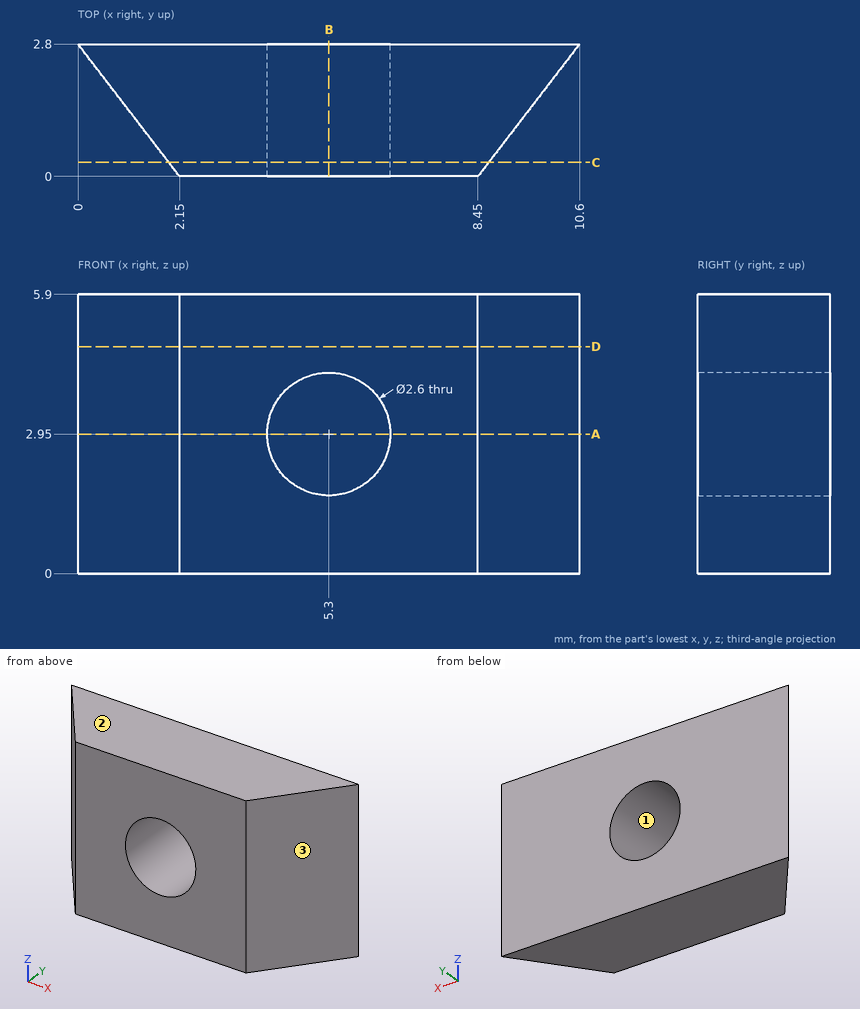
Geometry check sheet. Reference: drawing and pictorial views, mm from the part's lowest x, y, z. Coordinates: 2 decimals unless noted, no trailing zeros. Order: outer loops, then holes, each group sorted by start corner. A loop starts at its lowest first (then second) coordinate and runs counter-clockwise, first axis right, second up. Notation, with made-up numbers: (-10.5, -14.75) - (9.5, -14.75) arc R20 cw to (9.5, -6.75) - close; hole circle Ø2 at (40.25, 47). An arc over 180 degrees is marked (long way). Answer in a Markdown table with one row per item. Add a question column.
1) Cross-section at D-D, the plane z = 4.8. Record the cut outline in (x, y), then the cut area to 3 significant figures.
2) Cross-section at B-B, the plane x = 5.3. Record the cut outline in (y, z).
3) Cross-section at C-C, the plane y = 0.3. Record the cut outline in (x, z).
4) Release check for a two-part mould opening along X. For the marked faces 1, 2 and 3 record: +X half, -X half, draft (parallel to the pull), parting line (faces both ways), or undercut.
5) Cross-section at A-A, the plane z = 2.95. Record the cut outline in (x, y).
6) Material ranges on line 1 along X through (y, z) = (2.2, 2.95); line 2 along X through (y, z) = (0.8, 2.1); line 3 along Z through (x, y) = (5.75, 1.65), recorded low to high. Write a range as [from, to].
7) Gauge pin test, flat ends, axial feed: P1, Ø1.5, axis at y = 1.5, z = 3.5, coming from the +X side; P2, Ø1.6, axis at x = 5.3, z = 2.95, coming from the -Y side. Record the tip position at first contact, or that the pin passes through.
Check result:
| question | item | result |
|---|---|---|
| 1 | outline | (0, 2.8) - (2.15, 0) - (8.45, 0) - (10.6, 2.8) - close |
| 1 | area | 23.7 mm² |
| 2 | outline | (0, 0) - (2.8, 0) - (2.8, 1.65) - (0, 1.65) - close; (0, 4.25) - (2.8, 4.25) - (2.8, 5.9) - (0, 5.9) - close |
| 3 | outline | (1.92, 0) - (8.68, 0) - (8.68, 5.9) - (1.92, 5.9) - close; hole circle Ø2.6 at (5.3, 2.95) |
| 4 | face 1 | undercut |
| 4 | face 2 | draft |
| 4 | face 3 | +X half |
| 5 | outline | (0, 2.8) - (2.15, 0) - (4, 0) - (4, 2.8) - close; (6.6, 0) - (8.45, 0) - (10.6, 2.8) - (6.6, 2.8) - close |
| 6 | line 1 | x = [0.46, 4], [6.6, 10.14] |
| 6 | line 2 | x = [1.54, 4.32], [6.28, 9.06] |
| 6 | line 3 | z = [0, 1.73], [4.17, 5.9] |
| 7 | P1 | stops at x = 10.18 |
| 7 | P2 | passes through |
